Source: CAD feature listing. Evaluate the final solid. Frame: model axes, mm. Face numbers are marked on the shaded views. A direction names the side the tool comes from. Coordinates: 2 decimals unless noted, no trailing zeros. Loops run counter-clockwise (first coordinate to the right, second up) from the corner with the lowest first, then second, coordinate; pieces in that order, holes last.
Item 1: Section query D-D, the plane x = -0.5. Return the cut outline in (y, z).
Item 2: Section query C-C, the plane y = 1.5. Return the cut outline in (x, z).
Item 3: Section query A-A, the plane y = -1.75. Return the cut outline in (x, z), then the cut area to 3 significant figures.
Item 4: Reachability of the marked faces 1, 2, 3, 4 and 5 from +Z, -Z, +X, -X, +Y, -Y: full face, straight path, thin tool, end or side. Return the list, or none.
Item 5: Section query B-B, the plane z = -17.5. Return the cut outline in (x, y), then the cut area to 3 significant figures.
Item 6: Pin query (flat end, axial travel): pin 1 Ø1 at (x, z) = (-3, -6) entering from -Y; pin 2 Ø1.2 at (y, z) = (2.5, -6.5) entering from -X; pin 3 Ø0.6 at (x, z) = (-2, -15) entering from +Y; pin 4 Ø5.5 at (y, z) = (1.5, -17) entering from -X. Return the tip coordinate at first contact, or that it passes through.
Item 7: Pull-direction query (Z, two-part tool) for the marked faces 6, 7 and 8; classes: +Z half, -Z half, draft (parallel to the pull), parting line (faces both ways), or undercut.
Item 8: Line query: probe 1 along Y at (x, z) = (-3.75, -8.5); probe 2 along X at (y, z) = (7.75, -9); probe 3 along Y at (x, z) = (2, -9.75). Output: solid intervals per line, ascending.
```python
from build123d import *

# Parameters (mm, degrees)
BOSS_EXTRUDE1_DEPTH = 12.8
SKETCH2_W           = 1.14
SKETCH2_H           = 1.14
SKETCH4_W           = 1.14
SKETCH4_H           = 1.14
LPATTERN2_COUNT     = 2
LPATTERN2_PITCH     = 4.2
LPATTERN3_COUNT     = 2
LPATTERN3_PITCH     = 4.2
FILLET1_R           = 0.3
SKETCH6_W           = 4
SKETCH6_H           = 4
CUT_EXTRUDE1_DEPTH  = 12
SKETCH9_W           = 1.6
SKETCH9_H           = 3.5
CUT_EXTRUDE2_DEPTH  = 20.97


with BuildPart() as part:
    # Sketch1 → Boss-Extrude1 (new body)
    with BuildSketch(Plane.XY):
        Polygon((-4.5, 0.5), (-3.5, 0.5), (-3.5, 0), (-2.9, 0), (-2.9, 0.5), (2.9, 0.5), (2.9, 0), (3.5, 0), (3.5, 0.5), (4.5, 0.5), (4.5, 2.7), (4.9, 2.7), (4.9, 3.5), (4.5, 3.5), (4.5, 10.2), (-4.5, 10.2), (-4.5, 3.5), (-4.9, 3.5), (-4.9, 2.7), (-4.5, 2.7), align=None)
    extrude(amount=-BOSS_EXTRUDE1_DEPTH)

    # Sweep2: sweep along a path in Sketch3
    with BuildLine(Plane(origin=(2.1, 0, 0), x_dir=(0, 0, -1), z_dir=(1, 0, 0))) as sweep2_path:
        Line((12.8, 7.45), (18.4, 7.45))
        ThreePointArc((18.4, 7.45), (19.107106781, 7.157106781), (19.4, 6.45))
        Line((19.4, 6.45), (19.4, -1))
    # Sketch2 → Sweep2 (sweep)
    with BuildSketch(Plane(origin=(0, 0, -12.8), x_dir=(-1, 0, 0), z_dir=(0, 0, -1))):
        with Locations((-2.1, 7.45)):
            Rectangle(SKETCH2_W, SKETCH2_H)
    sweep2 = sweep(path=sweep2_path.line)

    # Sweep3: sweep along a path in Sketch5
    with BuildLine(Plane(origin=(2.1, 0, 0), x_dir=(0, 0, -1), z_dir=(1, 0, 0))) as sweep3_path:
        Line((12.8, 3.25), (12.9, 3.25))
        ThreePointArc((12.9, 3.25), (13.607106781, 2.957106781), (13.9, 2.25))
        Line((13.9, 2.25), (13.9, -1))
    # Sketch4 → Sweep3 (sweep)
    with BuildSketch(Plane(origin=(0, 0, -12.8), x_dir=(-1, 0, 0), z_dir=(0, 0, -1))):
        with Locations((-2.1, 3.25)):
            Rectangle(SKETCH4_W, SKETCH4_H)
    sweep3 = sweep(path=sweep3_path.line)

    # LPattern2: Sweep2 ×2
    with Locations(*[(-i * LPATTERN2_PITCH, 0, 0) for i in range(1, LPATTERN2_COUNT)]):
        add(sweep2)

    # LPattern3: Sweep3 ×2
    with Locations(*[(-i * LPATTERN3_PITCH, 0, 0) for i in range(1, LPATTERN3_COUNT)]):
        add(sweep3)

    # Fillet1
    fillet1_edges = [part.edges().sort_by_distance(p)[0] for p in [
        (-4.5, 10.2, -6.4),
        (4.5, 10.2, -6.4),
        (4.5, 0.5, -6.4),
        (-4.5, 0.5, -6.4),
    ]]
    fillet(fillet1_edges, radius=FILLET1_R)

    # Sketch6 → Cut-Extrude1 (cut)
    with BuildSketch(Plane.XY):
        Polygon((-4.2, 2.25), (-3.2, 1.25), (-1.2, 1.25), (-0.2, 2.25), (-0.2, 5.25), (-4.2, 5.25), align=None)
        with Locations((-2.2, 7.65)):
            Rectangle(SKETCH6_W, SKETCH6_H)
        with Locations((2.2, 3.25)):
            Rectangle(SKETCH6_W, SKETCH6_H)
        Polygon((0.2, 9.65), (4.2, 9.65), (4.2, 6.65), (3.2, 5.65), (1.2, 5.65), (0.2, 6.65), align=None)
    extrude(amount=-CUT_EXTRUDE1_DEPTH, mode=Mode.SUBTRACT)

    # Sketch8 → Revolve1 (revolve)
    with BuildSketch(Plane(origin=(0, 0, 0), x_dir=(0, 0, -1), z_dir=(1, 0, 0))):
        Polygon((5.6, 0.5), (5.6, -2.9), (5.150103769, -2.9), (4.8, -2.4), (5.1, -2.4), (5.1, 0.5), align=None)
    revolve(axis=Axis((0, 0.5, -6.6), (0, -1, 0)))

    # Sketch9 → Cut-Extrude2 (cut, through all)
    with BuildSketch(Plane.XY):
        with Locations((0, -1.25)):
            Rectangle(SKETCH9_W, SKETCH9_H)
    extrude(amount=-CUT_EXTRUDE2_DEPTH, mode=Mode.SUBTRACT)


solid = part.part
```
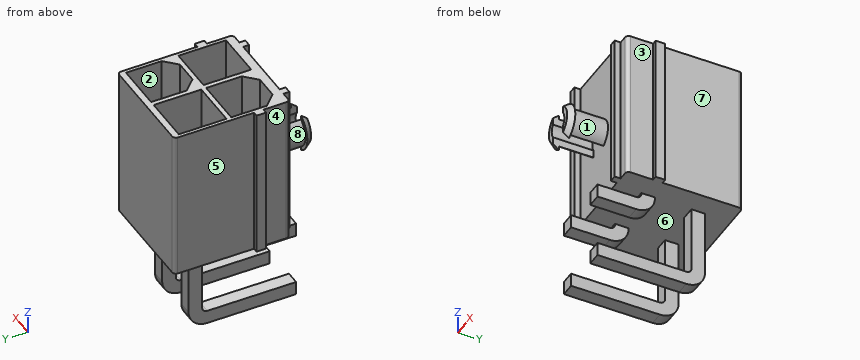
Verdict:
1. outline: (0.5, -12.8) - (10.2, -12.8) - (10.2, 0) - (9.65, 0) - (9.65, -12) - (5.65, -12) - (5.65, 0) - (5.25, 0) - (5.25, -12) - (1.95, -12) - (1.95, 0) - (0.5, 0) - close
2. outline: (-4.5, -12.8) - (4.5, -12.8) - (4.5, 0) - (4.2, 0) - (4.2, -12) - (0.2, -12) - (0.2, 0) - (-0.95, 0) - (-0.95, -12) - (-3.45, -12) - (-3.45, 0) - (-4.5, 0) - close; (-2.67, -19.97) - (-1.53, -19.97) - (-1.53, -18.83) - (-2.67, -18.83) - close; (-2.67, -14.47) - (-1.53, -14.47) - (-1.53, -13.33) - (-2.67, -13.33) - close; (1.53, -19.97) - (2.67, -19.97) - (2.67, -18.83) - (1.53, -18.83) - close; (1.53, -14.47) - (2.67, -14.47) - (2.67, -13.33) - (1.53, -13.33) - close
3. outline: (-0.8, -7.87) - (-0.8, -7.2) arc R1 cw to (-0.8, -6) - (-0.8, -5.33) arc R1.5 ccw to start; (0.8, -7.87) arc R1.5 ccw to (0.8, -5.33) - (0.8, -6) arc R1 cw to (0.8, -7.2) - close
3. area: 2.18 mm2
4. face 1: none
4. face 2: +Z
4. face 3: +Z, -Z, +X, -Y
4. face 4: +Z, -Z, -X, -Y
4. face 5: +Z, -Z, -X, +Y
5. outline: (-2.67, 6.88) - (-1.53, 6.88) - (-1.53, 8.02) - (-2.67, 8.02) - close; (1.53, 6.88) - (2.67, 6.88) - (2.67, 8.02) - (1.53, 8.02) - close
5. area: 2.60 mm2
6. pin 1: stops at y = 0
6. pin 2: stops at x = -4.9
6. pin 3: stops at y = 8.02
6. pin 4: stops at x = -2.67
7. face 6: undercut
7. face 7: draft
7. face 8: parting line
8. probe 1: y = 0.5 to 1.8, 5.25 to 5.65, 9.65 to 10.2
8. probe 2: x = -4.5 to -4.2, -0.2 to 0.2, 4.2 to 4.5
8. probe 3: y = 0.5 to 1.25, 5.25 to 5.65, 9.65 to 10.2
